Design review of the part built by this model. Coordinates are the model's own, in mm. A direction names the side the tool comes from. Coordinates: 2 decimals unless noted, no trailing zeros. Write each loop counter-clockwise with the first axis right and the second up, starting at its lowest first coordinate (ties: lowest second). Pieces come first, ordered by that corner, then holes.
Q1. The part is to be moulded in two halves that separate along X. For faces 3 (the flat face through (-26.803, 1, -15)), 4 (the flat face through (-31, 3, -15)), 5 (the flat face through (-30.733, 1.479, -16.684)), 6 (the flat face through (-31.982, 1, -13)), say which applies: released by +X, released by -X, zero draft, split by the parting line, or undercut.
Q2. For L1, parallel to X at y = 0.95, z = -12.5; L2, parallel to X at y = 0.9, z = -19.5; L3, parallel to X at y = 0.35, z = -16.75, list the stretches that pass through material, from the lowest coordinate up.
Q3. Take a section at A-A, the plane z = -13.75. Write out the cut boundary in (x, y), plus the area to 3 significant figures.
Q4. Take a section at B-B, the plane x = -30.25. Write out the cut boundary in (y, z), plus the area to 3 significant figures.
Q5. For faces 1 (the flat face through (-38.03, 1, -13)), 2 (the flat face through (-35, 1, -22.318)), list the 3-axis set-ups (+Z, -Z, +X, -X, +Y, -Y) from which the entire face can be reached by the end or side of a thin tool; tool diameter is ignored.
from build123d import *

# Parameters (mm, degrees)
SKETCH1_W           = 16
SKETCH1_H           = 14
BOSS_EXTRUDE1_DEPTH = 3


with BuildPart() as part:
    # Sketch1 → Boss-Extrude1 (new body)
    with BuildSketch(Plane(origin=(0, 0, 0), x_dir=(1, 0, 0), z_dir=(0, 1, 0))):
        with Locations((-34.802547771, 15.318471338)):
            Rectangle(SKETCH1_W, SKETCH1_H)
        with BuildLine():
            Line((-40.05451323, 17.459486991), (-38.524659604, 15.929633365))
            Line((-38.524659604, 15.929633365), (-38.030399201, 16.423893767))
            Line((-38.030399201, 16.423893767), (-38.030399201, 10.37508789))
            Line((-38.030399201, 10.37508789), (-31.981593325, 10.37508789))
            Line((-31.981593325, 10.37508789), (-31.981593325, 16.423893767))
            Line((-31.981593325, 16.423893767), (-31.487332922, 15.929633365))
            Line((-31.487332922, 15.929633365), (-29.957479296, 17.459486991))
            Line((-29.957479296, 17.459486991), (-31.734463123, 19.236470819))
            add(Edge.make_bspline(
                [(-31.734463123, 19.236470819), (-32.317966026, 19.664517133), (-32.090545187, 19.92760941), (-33.406999381, 19.883716584)],
                knots=[0, 0, 0, 0, 1, 1, 1, 1], degree=3))
            add(Edge.make_bspline(
                [(-36.594690414, 19.883716584), (-36.00950924, 18.767110628), (-34.074320208, 18.900131332), (-33.406999381, 19.883716584)],
                knots=[0, 0, 0, 0, 1, 1, 1, 1], degree=3))
            add(Edge.make_bspline(
                [(-38.277529403, 19.236470819), (-37.529085744, 19.813493214), (-36.594690414, 19.883716584)],
                knots=[0, 0, 0, 1, 1, 1], degree=2))
            Line((-38.277529403, 19.236470819), (-40.05451323, 17.459486991))
        make_face(mode=Mode.SUBTRACT)
    extrude(amount=BOSS_EXTRUDE1_DEPTH)


solid = part.part
Responses:
1. face 3: released by +X
1. face 4: zero draft
1. face 5: undercut
1. face 6: undercut
2. L1: x = -42.8 to -38.03, -31.98 to -26.8
2. L2: x = -42.8 to -37.88, -36.29 to -33.78, -32.03 to -26.8
2. L3: x = -42.8 to -39.35, -30.67 to -26.8
3. outline: (-42.8, 0) - (-38.03, 0) - (-38.03, 3) - (-42.8, 3) - close; (-31.98, 0) - (-26.8, 0) - (-26.8, 3) - (-31.98, 3) - close
3. area: 29.9 mm2
4. outline: (0, -22.32) - (3, -22.32) - (3, -17.75) - (0, -17.75) - close; (0, -17.17) - (3, -17.17) - (3, -8.32) - (0, -8.32) - close
4. area: 40.2 mm2
5. face 1: +Y, -Y
5. face 2: -Z, +X, -X, +Y, -Y
